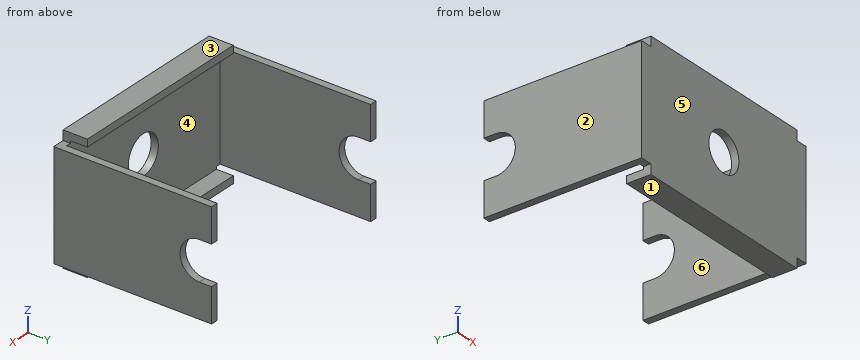
```python
from build123d import *

# Parameters (mm, degrees)
BOSS_EXTRUDE1_DEPTH = 11
BOSS_EXTRUDE2_DEPTH = 19.5
SKETCH3_R           = 4
CUT_EXTRUDE1_DEPTH  = 41.174618853
CUT_EXTRUDE2_DEPTH  = 57.224994442


with BuildPart() as part:
    # Sketch1 → Boss-Extrude1 (new, symmetric)
    with BuildSketch(Plane.XY):
        Polygon((-22, 32.5), (-22, 0), (22, 0), (22, 32.5), (20.5, 32.5), (20.5, 1.5), (-20.5, 1.5), (-20.5, 32.5), align=None)
    extrude(amount=BOSS_EXTRUDE1_DEPTH, both=True)

    # Sketch2 → Boss-Extrude2 (add, symmetric)
    with BuildSketch(Plane(origin=(0, 0, 0), x_dir=(0, 0, -1), z_dir=(1, 0, 0))):
        Polygon((-11, 0), (-13, 0), (-13, 5), (-11.5, 5), (-11.5, 1.5), (-11, 1.5), align=None)
    boss_extrude2 = extrude(amount=BOSS_EXTRUDE2_DEPTH, both=True)

    # Mirror1: Boss-Extrude2 across plane
    add(boss_extrude2.mirror(Plane.XY))

    # Sketch3 → Cut-Extrude1 (cut, through all)
    with BuildSketch(Plane(origin=(0, 1.5, 0), x_dir=(-1, 0, 0), z_dir=(0, 1, 0))):
        with Locations(Location((0, 0, 0), (0, 0, 90))):
            Circle(SKETCH3_R)
    extrude(amount=-CUT_EXTRUDE1_DEPTH, mode=Mode.SUBTRACT)

    # Sketch4 → Cut-Extrude2 (cut, through all)
    with BuildSketch(Plane(origin=(22, 0, 0), x_dir=(0, 0, -1), z_dir=(1, 0, 0))):
        with BuildLine():
            Line((-4, 30), (-4, 32.5))
            Line((-4, 32.5), (4, 32.5))
            Line((4, 32.5), (4, 30))
            ThreePointArc((4, 30), (0, 26), (-4, 30))
        make_face()
    extrude(amount=-CUT_EXTRUDE2_DEPTH, mode=Mode.SUBTRACT)


solid = part.part
```
Geometry: final body of the model. Coordinates: model frame, mm. Face numbers are marked on the shaded views. A direction names the side the tool comes from. Round coordinates to 2 decimals unless told otherwise and drop trailing zeros. Loops run counter-clockwise (first coordinate to the right, second up) from the corner with the lowest first, then second, coordinate; pieces in that order, holes last. Notation, with made-up numbers: (1, 11) -> (8, 11) arc R31 cw to (8, 44) -> close; hole circle Ø7 at (13, -39.75). An arc over 180 degrees is marked (long way). Use one line per item in the form item = value. Start each with the question number.
1) Section A-A on x = 0. Output: boundary loops of the cut face in (y, z).
2) Section C-C on y = 9. Output: boundary loops of the cut face in (x, z).
3) Access query for the marked faces 5 and 6. Directions: +Z, -Z, +X, -X, +Y, -Y. A direction counts if a zero-diameter tool reaches every point of the face in a straight line with its end or side. Return the directions, or none.
4) Section D-D on y = 28. Output: boundary loops of the cut face in (x, z).
5) Draft query along Z for the marked faces 1, 2, 3 and 4. Return one class per face: released by +Z, released by -Z, zero draft, split by the parting line, or undercut.
6) Line query: L1, parallel to X at y = 1.1, z = 0; L2, parallel to X at y = 18.5, z = -2.25; L3, parallel to Z at x = 7, y = 3. Output: solid intervals per line, ascending.
7) First-contact query: P1, Ø1.2, axis at x = 20.5, y = 9, coming from the -Z side; P2, Ø0.6, axis at y = 3, z = -12, coming from the +X side; P3, Ø0.8, axis at x = -21, y = 31.5, coming from the +Z side. Flat tips, straight axial feed; report the tip coordinate or a pass-through.
8) Section B-B on z = 0. Output: boundary loops of the cut face in (x, y), then the cut area to 4 significant figures.
Response:
q1.outline = (0, -13) -> (5, -13) -> (5, -11.5) -> (1.5, -11.5) -> (1.5, -4) -> (0, -4) -> close; (0, 4) -> (1.5, 4) -> (1.5, 11.5) -> (5, 11.5) -> (5, 13) -> (0, 13) -> close
q2.outline = (-22, -11) -> (-20.5, -11) -> (-20.5, 11) -> (-22, 11) -> close; (20.5, -11) -> (22, -11) -> (22, 11) -> (20.5, 11) -> close
q3.face_5 = +Z, -Z, +X, -X, -Y
q3.face_6 = +Z, -Z, +Y
q4.outline = (-22, -11) -> (-20.5, -11) -> (-20.5, -3.46) -> (-22, -3.46) -> close; (-22, 3.46) -> (-20.5, 3.46) -> (-20.5, 11) -> (-22, 11) -> close; (20.5, -11) -> (22, -11) -> (22, -3.46) -> (20.5, -3.46) -> close; (20.5, 3.46) -> (22, 3.46) -> (22, 11) -> (20.5, 11) -> close
q5.face_1 = released by -Z
q5.face_2 = zero draft
q5.face_3 = released by +Z
q5.face_4 = undercut
q6.L1 = -22 to -4, 4 to 22
q6.L2 = -22 to -20.5, 20.5 to 22
q6.L3 = -13 to -11.5, 11.5 to 13
q7.P1 = -11
q7.P2 = 19.5
q7.P3 = 11
q8.outline = (-22, 0) -> (-4, 0) -> (-4, 1.5) -> (-20.5, 1.5) -> (-20.5, 26) -> (-22, 26) -> close; (4, 0) -> (22, 0) -> (22, 26) -> (20.5, 26) -> (20.5, 1.5) -> (4, 1.5) -> close
q8.area = 127.5 mm^2
